Could you check a few things on this model? Use its own coordinates, in mm. A direction names the side the tool comes from. Give positions to 0.01 mm unless a question says otherwise; leave off trailing zeros. Write each loop counter-clockwise with the first axis right and the second up, starting at its lowest first coordinate (ties: lowest second). Pieces come first, ordered by that corner, then holes. Notation, with made-up numbers: (-26, 70.25) - (22, 70.25) arc R20 ccw to (22, 80.25) - close; hole circle Ø11 at (35.25, 56.25). An arc over 180 degrees is marked (long way). Use one line per item in the form item = value.
Autodesk Inventor part; units mm, degrees
ref_plane "YZ Plane" through (0, 0, 0) normal (1, 0, 0) x (0, 1, 0)
ref_plane "XZ Plane" through (0, 0, 0) normal (0, 1, 0) x (-1, 0, 0)
ref_plane "XY Plane" through (0, 0, 0) normal (0, 0, 1) x (1, 0, 0)
sketch "スケッチ1" plane through (0, 0, 0) normal (0, 0, 1) x (1, 0, 0)
  circle A0 centre (0, 0) radius 5
  circle A1 centre (0, 0) radius 8.5
  dimension "d0" = 10
  dimension "d1" = 17
extrude "押し出し1" add sketch "スケッチ1" along normal blind 0.5
sketch "スケッチ2" plane through (0, 0, 0.5) normal (0, 0, 1) x (1, 0, 0)
  circle A0 centre (0, 0) radius 7.5
  dimension "d4" = 15
extrude "押し出し2" add sketch "スケッチ2" along normal blind 3
sketch "スケッチ3" plane through (0, 0, 3.5) normal (0, 0, 1) x (1, 0, 0)
  circle A0 centre (0, 0) radius 5
  dimension "d7" = 10
extrude "押し出し3" cut sketch "スケッチ3" against normal blind 5
properties part number "bearing10-15"
1. If I drill on line 1 (Y direction, x = 0, z = 0.85); line 2 (X direction, y = -1, z = 0.4); line 3 (X direction, y = -1, z = 2.6), over which ranges is the centre line in solid material (lowest first)? Write a range as from..to.
Response values:
line_1 = -7.5..-5, 5..7.5
line_2 = -8.44..-4.9, 4.9..8.44
line_3 = -7.43..-4.9, 4.9..7.43
2. If we mould it in two halves opening along Y, with no side actions, what happens to faces 3 (the face through (-1.08, 4.88, 1.73)), 4 (the face through (4, -4, 0)), 5 (the face through (4.57, -7.167, 0.246))? For each: pulls with the +Y half, pulls with the -Y half, needs draft (parallel to the pull), parting line crosses it, or undercut.
Response values:
face_3 = undercut
face_4 = needs draft
face_5 = parting line crosses it
3. Imagine slicing it at D-D, the plane x = -5.75. List the corners of the cut face in (y, z) for me.
Response values:
outline = (-6.26, 0) - (6.26, 0) - (6.26, 0.5) - (4.82, 0.5) - (4.82, 3.5) - (-4.82, 3.5) - (-4.82, 0.5) - (-6.26, 0.5) - close
4. For pin 1 (2 mm diameter, centred on y = 2, z = 2, fed in from +X); pin 2 (2 mm diameter, centred on x = -0.5, z = 2, fed in from +Y); pin 3 (2 mm diameter, centred on x = -3.5, z = 2.5, fed in from -Y), each with a flat end and sliding along its axis, tell me the tip position at first contact or that it passes through.
Response values:
pin_1 = 7.43
pin_2 = 7.5
pin_3 = -7.07
5. Which directions (+Z, -Z, +X, -X, +Y, -Y) give clear straight access to the entire face, cutting with the end or side of a thin tool? Please do faces 1 (the face through (0, -8, 0.5)), 2 (the face through (2, -5, 3.5)).
Response values:
face_1 = +Z
face_2 = +Z, +X, -X, +Y, -Y
6. Imagine slicing it at C-C, the plane z = 3.25. List the corners of the cut face in (x, y) for me.
Response values:
outline = circle Ø15 at (0, 0); hole circle Ø10 at (0, 0)
7. Imagine slicing it at A-A, the plane y = 0. List the corners of the cut face in (x, z) for me, and give its area (3 significant figures).
Response values:
outline = (-8.5, 0) - (-5, 0) - (-5, 3.5) - (-7.5, 3.5) - (-7.5, 0.5) - (-8.5, 0.5) - close; (5, 0) - (8.5, 0) - (8.5, 0.5) - (7.5, 0.5) - (7.5, 3.5) - (5, 3.5) - close
area = 18.5 mm²
